The model under review builds one solid part; all positions refer to its coordinate system, in mm. A direction names the side the tool comes from. Coordinates: 2 decimals unless noted, no trailing zeros. Order: outer loops, then holes, each group sorted by start corner. A loop starts at its lowest first (then second) coordinate and runs counter-clockwise, first axis right, second up. Notation, with made-up numbers: (73.25, -23.75) - (118.25, -23.75) arc R22 ccw to (118.25, -3.75) - close; hole circle Ø7 at (74, 27). An arc over 180 degrees is marked (long way). Answer in a Markdown table with one row per item.
```python
from build123d import *

# Parameters (mm, degrees)
F0_W      = 190
F0_H      = 90
F0_R      = 1.75
F0_R_2    = 5.5
F0_W_2    = 79.652223
F0_H_2    = 18.950621
F1_DEPTH  = 8
F2_R      = 5
F4_DEPTH  = 4
F5_SIZE   = 0.5
F6_SIZE   = 1
F7_R      = 2
F8_R      = 2.8
F9_DEPTH  = 3
F11_DEPTH = 5.5
F12_R     = 1.75
F13_DEPTH = 1.6


with BuildPart() as f1:
    # F0 (on Top) → F1 (new body)
    with BuildSketch(Plane.XY):
        Rectangle(F0_W, F0_H)
        with Locations((-87, -37)):
            Circle(F0_R, mode=Mode.SUBTRACT)
        with Locations((-62.5, -30.559658)):
            Circle(F0_R_2, mode=Mode.SUBTRACT)
        with Locations((87, -37)):
            Circle(F0_R, mode=Mode.SUBTRACT)
        with Locations((-62.5, 3.348534)):
            Circle(F0_R_2, mode=Mode.SUBTRACT)
        with Locations((-74.5, 15.348534)):
            Circle(F0_R_2, mode=Mode.SUBTRACT)
        with Locations((-50.5, 15.348534)):
            Circle(F0_R_2, mode=Mode.SUBTRACT)
        with Locations((-62.5, 27.348534)):
            Circle(F0_R_2, mode=Mode.SUBTRACT)
        with Locations((-87, 37)):
            Circle(F0_R, mode=Mode.SUBTRACT)
        with Locations((8.005532, 15.213479)):
            Rectangle(F0_W_2, F0_H_2, mode=Mode.SUBTRACT)
        with Locations((72.103191, 6.74016)):
            Circle(F0_R_2, mode=Mode.SUBTRACT)
        with Locations((72.144568, 22.672617)):
            Circle(F0_R_2, mode=Mode.SUBTRACT)
        with Locations((87, 37)):
            Circle(F0_R, mode=Mode.SUBTRACT)
    extrude(amount=F1_DEPTH)

    # F2
    f2_edges = [f1.edges().sort_by_distance(p)[0] for p in [
        (-95, 45, 4),
        (-95, -45, 4),
        (95, -45, 4),
        (95, 45, 4),
    ]]
    fillet(f2_edges, radius=F2_R)

    # F3 (on face) → F4 (cut)
    with BuildSketch(Plane(origin=(0, 0, 0), x_dir=(1, 0, 0), z_dir=(0, 0, -1))):
        with BuildLine():
            ThreePointArc((82.417424, -39), (83.464466, -33.464466), (89, -32.417424))
            Line((89, -32.417424), (89, 32.417424))
            ThreePointArc((89, 32.417424), (83.464466, 33.464466), (82.417424, 39))
            Line((82.417424, 39), (-82.417424, 39))
            ThreePointArc((-82.417424, 39), (-83.464466, 33.464466), (-89, 32.417424))
            Line((-89, 32.417424), (-89, -32.417424))
            ThreePointArc((-89, -32.417424), (-83.464466, -33.464466), (-82.417424, -39))
            Line((-82.417424, -39), (82.417424, -39))
        make_face()
    extrude(amount=-F4_DEPTH, mode=Mode.SUBTRACT)

    # F5
    f5_edges = [f1.edges().sort_by_distance(p)[0] for p in [
        (-68, 27.348534, 8),
        (-56, 15.348534, 8),
        (-80, 15.348534, 8),
        (-68, 3.348534, 8),
        (-68, -30.559658, 8),
        (66.644568, 22.672617, 8),
        (66.603191, 6.74016, 8),
    ]]
    chamfer(f5_edges, length=F5_SIZE)

    # F6
    f6_edges = [f1.edges().sort_by_distance(p)[0] for p in [
        (8.005532, 24.688789, 8),
        (-31.82058, 15.213478, 8),
        (47.831643, 15.213478, 8),
        (8.005532, 5.738168, 8),
        (0, 45, 8),
    ]]
    chamfer(f6_edges, length=F6_SIZE)

    # F7
    f7_edges = [f1.edges().sort_by_distance(p)[0] for p in [
        (-89, -32.417424, 2),
        (-82.417424, -39, 2),
        (82.417424, -39, 2),
        (89, -32.417424, 2),
        (89, 32.417424, 2),
        (82.417424, 39, 2),
        (-82.417424, 39, 2),
        (-89, 32.417424, 2),
    ]]
    fillet(f7_edges, radius=F7_R)

    # F8 (on face) → F9 (cut)
    with BuildSketch(Plane.XY.offset(8)):
        with Locations((-87, 37)):
            Circle(F8_R)
        with Locations((87, 37)):
            Circle(F8_R)
        with Locations((-87, -37)):
            Circle(F8_R)
        with Locations((87, -37)):
            Circle(F8_R)
    extrude(amount=-F9_DEPTH, mode=Mode.SUBTRACT)

    # F10 (on face) → F11 (cut)
    with BuildSketch(Plane(origin=(0, 0, 0), x_dir=(1, 0, 0), z_dir=(0, 0, -1))):
        with BuildLine():
            Line((-90, -45), (90, -45))
            ThreePointArc((90, -45), (93.535534, -43.535534), (95, -40))
            Line((95, -40), (95, 40))
            ThreePointArc((95, 40), (93.535534, 43.535534), (90, 45))
            Line((90, 45), (-90, 45))
            ThreePointArc((-90, 45), (-93.535534, 43.535534), (-95, 40))
            Line((-95, 40), (-95, -40))
            ThreePointArc((-95, -40), (-93.535534, -43.535534), (-90, -45))
        make_face()
        with BuildLine():
            ThreePointArc((92.5, -40), (91.767767, -41.767767), (90, -42.5))
            Line((90, -42.5), (-90, -42.5))
            ThreePointArc((-90, -42.5), (-91.767767, -41.767767), (-92.5, -40))
            Line((-92.5, -40), (-92.5, 40))
            ThreePointArc((-92.5, 40), (-91.767767, 41.767767), (-90, 42.5))
            Line((-90, 42.5), (90, 42.5))
            ThreePointArc((90, 42.5), (91.767767, 41.767767), (92.5, 40))
            Line((92.5, 40), (92.5, -40))
        make_face(mode=Mode.SUBTRACT)
    extrude(amount=-F11_DEPTH, mode=Mode.SUBTRACT)

    # F12 (on face) → F13 (join)
    with BuildSketch(Plane(origin=(0, 0, 0), x_dir=(1, 0, 0), z_dir=(0, 0, -1))):
        with BuildLine():
            Line((90, 42), (-90, 42))
            ThreePointArc((-90, 42), (-91.414214, 41.414214), (-92, 40))
            Line((-92, 40), (-92, -40))
            ThreePointArc((-92, -40), (-91.414214, -41.414214), (-90, -42))
            Line((-90, -42), (90, -42))
            ThreePointArc((90, -42), (91.414214, -41.414214), (92, -40))
            Line((92, -40), (92, 40))
            ThreePointArc((92, 40), (91.414214, 41.414214), (90, 42))
        make_face()
        with Locations((-87, -37)):
            Circle(F12_R, mode=Mode.SUBTRACT)
        with Locations((87, -37)):
            Circle(F12_R, mode=Mode.SUBTRACT)
        with Locations((-87, 37)):
            Circle(F12_R, mode=Mode.SUBTRACT)
        with Locations((87, 37)):
            Circle(F12_R, mode=Mode.SUBTRACT)
    extrude(amount=F13_DEPTH)


solid = f1.part
```
Item 1: Mouldability with a two-part tool opening along X and no side actions: class faces 1 (the face through (-85.383, 37.67, 1.746)), 2 (the face through (93.063, -42.996, 7.715)), 3 (the face through (-1, -1, -1.6)) as +X half, -X half, draft (parallel to the pull), parting line (faces both ways), or undercut.
Check values:
| item | result |
|---|---|
| face 1 | undercut |
| face 2 | +X half |
| face 3 | draft |
Item 2: We need section A-A, the plane x = 42. Write out the cut boundary in (y, z), then the cut area to 3 significant figures.
Check values:
| item | result |
|---|---|
| outline | (-45, 5.5) - (-42.5, 5.5) - (-42.5, 0) - (-42, 0) - (-42, -1.6) - (42, -1.6) - (42, 0) - (42.5, 0) - (42.5, 5.5) - (45, 5.5) - (45, 7) - (44, 8) - (25.69, 8) - (24.69, 7) - (24.69, 4) - (39, 4) - (39, 0) - (-39, 0) - (-39, 4) - (5.74, 4) - (5.74, 7) - (4.74, 8) - (-44, 8) - (-45, 7) - close |
| area | 437 mm^2 |
Item 3: Tool access review of faces 4 (the face through (-84, 33, 2)), 5 (the face through (88.617, 37.67, 1.746)), 6 (the face through (77.225, 20.566, 5.726)): name each direction out of +Z, -Z, +X, -X, +Y, -Y from which nothing blocks a thin tool from reaching the whole face with its end or side.
Check values:
| item | result |
|---|---|
| face 4 | none |
| face 5 | +Z, -Z |
| face 6 | +Z |
Item 4: Clearance check with flat-ended pins moving along their axes: pin 1 Ø1.7 at (x, y) = (88.5, -36) entering from +Z; pin 2 Ø0.8 at (x, z) = (-3.5, -0.5) entering from -Y; pin 3 Ø0.9 at (y, z) = (19.5, 5) entering from +X. State where each tip first meets the part, or that it passes through.
Check values:
| item | result |
|---|---|
| pin 1 | z = 5 |
| pin 2 | y = -42 |
| pin 3 | x = 92.5 |
Item 5: We need section B-B, the plane x = -50.5. Write out the cut boundary in (y, z), then the cut area to 3 significant figures.
Check values:
| item | result |
|---|---|
| outline | (-45, 5.5) - (-42.5, 5.5) - (-42.5, 0) - (-42, 0) - (-42, -1.6) - (42, -1.6) - (42, 0) - (42.5, 0) - (42.5, 5.5) - (45, 5.5) - (45, 7) - (44, 8) - (21.35, 8) - (20.85, 7.5) - (20.85, 4) - (39, 4) - (39, 0) - (-39, 0) - (-39, 4) - (9.85, 4) - (9.85, 7.5) - (9.35, 8) - (-44, 8) - (-45, 7) - close |
| area | 470 mm^2 |
Item 6: To check wall thickness, follow line 1 (Y direction, x = -87, z = 3.5); line 2 (Z direction, x = 59.5, y = -36.5); line 3 (X direction, y = -26, z = 2). State the ranges of each line that lie inside material, in increasing order. Write a range as from..to.
Check values:
| item | result |
|---|---|
| line 1 | -42.5..-38.75, -35.25..-32, 32..35.25, 38.75..42.5 |
| line 2 | -1.6..0, 4..8 |
| line 3 | -92.5..-89, 89..92.5 |
